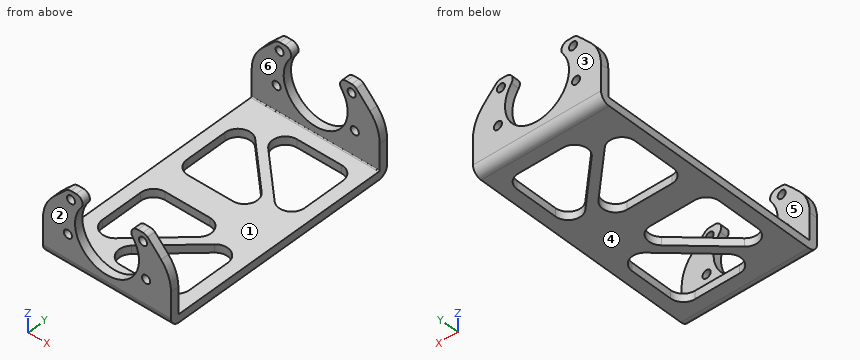
from build123d import *

# Parameters (mm, degrees)
SKETCH1_W                    = 100
SKETCH1_H                    = 60
BASE_FLANGE1_DEPTH           = 6.35
EDGE_FLANGE2_STRIP_W         = 26.8732
EDGE_FLANGE2_STRIP_H         = 6.35
EDGE_FLANGE2_STRIP_CUT_DEPTH = 100
EDGE_FLANGE2_DEPTH           = 100
EDGE_FLANGE3_STRIP_W         = 26.8732
EDGE_FLANGE3_STRIP_H         = 6.35
EDGE_FLANGE3_STRIP_CUT_DEPTH = 100
EDGE_FLANGE3_DEPTH           = 100
SKETCH27_R                   = 25
CUT_EXTRUDE2_DEPTH           = 196.975534187
FILLET3_R                    = 5
F_1_4_0_25_DIAMETER_HOLE1_D  = 6.35
CUT_EXTRUDE3_DEPTH           = 203.74715781
CUT_EXTRUDE4_DEPTH           = 196.975534187
FILLET4_R                    = 30
FILLET5_R                    = 5


# Sheet-metal steps are written as plain solids
with BuildPart() as part:
    # Sketch1 → Base-Flange1 (new body)
    with BuildSketch(Plane(origin=(0, 0, 0), x_dir=(1, 0, 0), z_dir=(0, 1, 0))):
        Rectangle(SKETCH1_W, SKETCH1_H)
    extrude(amount=-BASE_FLANGE1_DEPTH)

    # Edge-Flange2 strip (across the edge) → Edge-Flange2 strip cut (cut)
    with BuildSketch(Plane(origin=(-50, -6.35, -30), x_dir=(0, 0, 1), z_dir=(1, 0, 0))):
        with Locations((-6.35, -3.175)):
            Rectangle(EDGE_FLANGE2_STRIP_W, EDGE_FLANGE2_STRIP_H)
    extrude(amount=EDGE_FLANGE2_STRIP_CUT_DEPTH, mode=Mode.SUBTRACT)

    # Edge-Flange2 section (across the edge) → Edge-Flange2 (add)
    with BuildSketch(Plane(origin=(-50, -6.35, -30), x_dir=(0, 0, 1), z_dir=(1, 0, 0))):
        with BuildLine():
            Line((0, 0.7366), (0, 180.75))
            Line((0, 180.75), (6.35, 180.75))
            Line((6.35, 180.75), (6.35, 0.7366))
            ThreePointArc((6.35, 0.7366), (6.565745145, 0.215745145), (7.0866, 0))
            Line((7.0866, 0), (7.0866, -6.35))
            ThreePointArc((7.0866, -6.35), (2.075617084, -4.274382916), (0, 0.7366))
        make_face()
    extrude(amount=EDGE_FLANGE2_DEPTH)

    # Edge-Flange3 strip (across the edge) → Edge-Flange3 strip cut (cut)
    with BuildSketch(Plane(origin=(-50, -187.1, -23.65), x_dir=(0, 1, 0), z_dir=(1, 0, 0))):
        with Locations((-6.35, -3.175)):
            Rectangle(EDGE_FLANGE3_STRIP_W, EDGE_FLANGE3_STRIP_H)
    extrude(amount=EDGE_FLANGE3_STRIP_CUT_DEPTH, mode=Mode.SUBTRACT)

    # Edge-Flange3 section (across the edge) → Edge-Flange3 (add)
    with BuildSketch(Plane(origin=(-50, -187.1, -23.65), x_dir=(0, 1, 0), z_dir=(1, 0, 0))):
        with BuildLine():
            Line((0, 0.7366), (0, 53.65))
            Line((0, 53.65), (6.35, 53.65))
            Line((6.35, 53.65), (6.35, 0.7366))
            ThreePointArc((6.35, 0.7366), (6.565745145, 0.215745145), (7.0866, 0))
            Line((7.0866, 0), (7.0866, -6.35))
            ThreePointArc((7.0866, -6.35), (2.075617084, -4.274382916), (0, 0.7366))
        make_face()
    extrude(amount=EDGE_FLANGE3_DEPTH)

    # Sketch27 → Cut-Extrude2 (cut, through all)
    with BuildSketch(Plane.XZ.offset(187.1)):
        with Locations((0, 7.0866)):
            Circle(SKETCH27_R)
    extrude(amount=-CUT_EXTRUDE2_DEPTH, mode=Mode.SUBTRACT)

    # Fillet3
    fillet3_edges = [part.edges().sort_by_distance(p)[0] for p in [
        (-50, -183.925, 30),
        (50, -183.925, 30),
        (50, -3.175, 30),
        (-50, -3.175, 30),
        (9.998804951, -183.925, 30),
        (-9.998804951, -183.925, 30),
        (-9.998804951, -3.175, 30),
        (9.998804951, -3.175, 30),
    ]]
    fillet(fillet3_edges, radius=FILLET3_R)

    # 1/4 (0.25) Diameter Hole1 (through all)
    with Locations(Plane(origin=(0, 0, 0), x_dir=(1, 0, 0), z_dir=(0, 1, 0))):
        with Locations((28.145825623, -23.3366), (-30.540010176, 4.029054658), (30.540010176, 4.029054658), (-28.145825623, -23.3366)):
            Hole(F_1_4_0_25_DIAMETER_HOLE1_D / 2)

    # Sketch30 → Cut-Extrude3 (cut, through all)
    with BuildSketch(Plane(origin=(0, 0, -30), x_dir=(-1, 0, 0), z_dir=(0, 0, -1))):
        with BuildLine():
            Line((-40, -27.0866), (-40, -60.265715002))
            ThreePointArc((-40, -60.265715002), (-33.94619985, -69.454159198), (-23.114498651, -67.517602423))
            Line((-23.114498651, -67.517602423), (11.830118238, -34.338487421))
            ThreePointArc((11.830118238, -34.338487421), (14.232212762, -23.379773474), (4.944616889, -17.0866))
            Line((4.944616889, -17.0866), (-30, -17.0866))
            ThreePointArc((-30, -17.0866), (-37.071067812, -20.015532188), (-40, -27.0866))
        make_face()
        with BuildLine():
            Line((23.114498651, -33.118997577), (-11.830118238, -66.298112579))
            ThreePointArc((-11.830118238, -66.298112579), (-14.232212762, -77.256826526), (-4.944616889, -83.55))
            Line((-4.944616889, -83.55), (30, -83.55))
            ThreePointArc((30, -83.55), (37.071067812, -80.621067812), (40, -73.55))
            Line((40, -73.55), (40, -40.370884998))
            ThreePointArc((40, -40.370884998), (33.94619985, -31.182440802), (23.114498651, -33.118997577))
        make_face()
        with BuildLine():
            Line((-23.114498651, -119.582397577), (11.830118238, -152.761512579))
            ThreePointArc((11.830118238, -152.761512579), (14.232212762, -163.720226526), (4.944616889, -170.0134))
            Line((4.944616889, -170.0134), (-30, -170.0134))
            ThreePointArc((-30, -170.0134), (-37.071067812, -167.084467812), (-40, -160.0134))
            Line((-40, -160.0134), (-40, -126.834284998))
            ThreePointArc((-40, -126.834284998), (-33.94619985, -117.645840802), (-23.114498651, -119.582397577))
        make_face()
        with BuildLine():
            Line((-4.944616889, -103.55), (30, -103.55))
            ThreePointArc((30, -103.55), (37.071067812, -106.478932188), (40, -113.55))
            Line((40, -113.55), (40, -146.729115002))
            ThreePointArc((40, -146.729115002), (33.94619985, -155.917559198), (23.114498651, -153.981002423))
            Line((23.114498651, -153.981002423), (-11.830118238, -120.801887421))
            ThreePointArc((-11.830118238, -120.801887421), (-14.232212762, -109.843173474), (-4.944616889, -103.55))
        make_face()
    extrude(amount=-CUT_EXTRUDE3_DEPTH, mode=Mode.SUBTRACT)

    # Sketch31 → Cut-Extrude4 (cut, through all)
    with BuildSketch(Plane.XZ.offset(187.1)):
        with BuildLine():
            Line((30.246393456, 30), (50, 30))
            Line((50, 30), (50, 8.486121202))
            ThreePointArc((50, 8.486121202), (40.425530077, 19.520656941), (30.246393456, 30))
        make_face()
        with BuildLine():
            Line((-30.246393456, 30), (-50, 30))
            Line((-50, 30), (-50, 8.486121202))
            ThreePointArc((-50, 8.486121202), (-40.425530077, 19.520656941), (-30.246393456, 30))
        make_face()
    extrude(amount=-CUT_EXTRUDE4_DEPTH, mode=Mode.SUBTRACT)

    # Fillet4
    fillet4_edges = [part.edges().sort_by_distance(p)[0] for p in [
        (50, -3.175, 8.486121202),
        (50, -183.925, 8.486121202),
        (-50, -3.175, 8.486121202),
        (-50, -183.925, 8.486121202),
    ]]
    fillet(fillet4_edges, radius=FILLET4_R)

    # Fillet5
    fillet5_edges = [part.edges().sort_by_distance(p)[0] for p in [
        (30.246393456, -3.175, 30),
        (30.246393456, -183.925, 30),
        (-30.246393456, -3.175, 30),
        (-30.246393456, -183.925, 30),
    ]]
    fillet(fillet5_edges, radius=FILLET5_R)


solid = part.part
Verification items for the finished model (mm, model axes). Face numbers are marked on the shaded views. A direction names the side the tool comes from. Round coordinates to 2 decimals unless told otherwise and drop trailing zeros. Order: outer loops, then holes, each group sorted by start corner. A loop starts at its lowest first (then second) coordinate and runs counter-clockwise, first axis right, second up. Notation, with made-up numbers: (22, 54) -> (58, 54) arc R18 cw to (58, 65) -> close; hole circle Ø10 at (-6.75, 55). An arc over 180 degrees is marked (long way). Put each result on its own line as item: value.
1) Set-up check for the marked faces 1 and 2: record each of +Z, -Z, +X, -X, +Y, -Y from which the full face is reachable in a straight line by a thin tool's end or side.
Final values:
face 1: +Z, +X, -X
face 2: +Z, -Z, +X, -X, -Y
2) Section check B-B (y = -109). Record the cut outline in (x, z), then the cut area to 3 significant figures.
Final values:
outline: (-50, -30) -> (-38.9, -30) -> (-38.9, -23.65) -> (-50, -23.65) -> close; (13.85, -30) -> (50, -30) -> (50, -23.65) -> (13.85, -23.65) -> close
area: 300 mm^2
3) Mould release check, pull along Y, two halves, no side actions. Record for the marked faces 3, 4, 5 and 6: +Y half, -Y half, draft (parallel to the pull), parting line (faces both ways), or undercut.
Final values:
face 3: +Y half
face 4: draft
face 5: undercut
face 6: undercut
4) Material ranges on line 1 (Y direction, x = -35, z = -26); line 2 (X direction, y = -160, z = -26); line 3 (Y direction, x = 19, z = -16), recorded low to high.
Final values:
line 1: y = -186.39 to -155.39, -104.89 to -82.21, -31.71 to -0.71
line 2: x = -50 to -14.94, 40 to 50
line 3: y = -187.1 to -180.75, -6.35 to 0
5) Depth check by flat-ended pin: pin 1 (5 mm diameter, centred on x = 21, z = -28, fed in from +Y); pin 2 (1.9 mm diameter, centred on x = -17, z = -25.5, fed in from -Y). Enter the tip coordinate at first touch or a pass-through.
Final values:
pin 1: stops at y = -0.49
pin 2: stops at y = -186.91
6) Section check A-A (z = 13.5). Record the cut outline in (x, y), then the cut area to 3 significant figures.
Final values:
outline: (-45.31, -187.1) -> (-24.16, -187.1) -> (-24.16, -180.75) -> (-45.31, -180.75) -> close; (-45.31, -6.35) -> (-24.16, -6.35) -> (-24.16, 0) -> (-45.31, 0) -> close; (24.16, -187.1) -> (45.31, -187.1) -> (45.31, -180.75) -> (24.16, -180.75) -> close; (24.16, -6.35) -> (45.31, -6.35) -> (45.31, 0) -> (24.16, 0) -> close
area: 537 mm^2
7) Section check C-C (x = 0). Record the cut outline in (y, z).
Final values:
outline: (-187.1, -22.91) arc R7.09 ccw to (-180.01, -30) -> (-170.01, -30) -> (-170.01, -23.65) -> (-180.01, -23.65) arc R0.74 cw to (-180.75, -22.91) -> (-180.75, -17.91) -> (-187.1, -17.91) -> close; (-141.53, -30) -> (-132.03, -30) -> (-132.03, -23.65) -> (-141.53, -23.65) -> close; (-103.55, -30) -> (-83.55, -30) -> (-83.55, -23.65) -> (-103.55, -23.65) -> close; (-55.07, -30) -> (-45.57, -30) -> (-45.57, -23.65) -> (-55.07, -23.65) -> close; (-17.09, -30) -> (-7.09, -30) arc R7.09 ccw to (0, -22.91) -> (0, -17.91) -> (-6.35, -17.91) -> (-6.35, -22.91) arc R0.74 cw to (-7.09, -23.65) -> (-17.09, -23.65) -> close
8) Section check D-D (x = -38). Record the cut outline in (y, z), then the cut area to 3 significant figures.
Final values:
outline: (-187.1, -22.91) arc R7.09 ccw to (-180.01, -30) -> (-152.73, -30) -> (-152.73, -23.65) -> (-180.01, -23.65) arc R0.74 cw to (-180.75, -22.91) -> (-180.75, 22.13) -> (-187.1, 22.13) -> close; (-107.55, -30) -> (-79.55, -30) -> (-79.55, -23.65) -> (-107.55, -23.65) -> close; (-34.37, -30) -> (-7.09, -30) arc R7.09 ccw to (0, -22.91) -> (0, 22.13) -> (-6.35, 22.13) -> (-6.35, -22.91) arc R0.74 cw to (-7.09, -23.65) -> (-34.37, -23.65) -> close
area: 1,170 mm^2
